from build123d import *

# Parameters (mm, degrees)
PAD_DEPTH = 10


with BuildPart() as part:
    # Sketch → Pad (new body)
    with BuildSketch(Plane.XY):
        with BuildLine():
            ThreePointArc((2.5, 0), (0, 2.5), (-2.5, 0))
            Line((-2.5, 0), (-2.5, -10))
            ThreePointArc((-2.5, -10), (0, -12.5), (2.5, -10))
            Line((2.5, -7.625), (2.5, -10))
            Line((7.5, -7.625), (2.5, -7.625))
            Line((7.5, -2.375), (7.5, -7.625))
            Line((2.5, -2.375), (7.5, -2.375))
            Line((2.5, 0), (2.5, -2.375))
        make_face()
    extrude(amount=PAD_DEPTH)


solid = part.part
Geometry: final body of the model. Coordinates: model frame, mm. A direction names the side the tool comes from. Give positions to 0.01 mm unless a question says otherwise; leave off trailing zeros. Write each loop counter-clockwise with the first axis right and the second up, starting at its lowest first coordinate (ties: lowest second). Pieces come first, ordered by that corner, then holes.
(1) First-contact query: P1, Ø2.5, axis at y = -1, z = 3.5, coming from the +X side; P2, Ø5.5, axis at x = 4, z = 4, coming from the -Y side; P3, Ø1, axis at y = 1, z = 3.5, coming from the -X side. Flat tips, straight axial feed; report the tip coordinate or a pass-through.
(2) Mould query, pull axis X, two halves, no side actions, for faces 4 (the flat face through (5, -2.375, 5)), 5 (the flat face through (2.5, -9, 5)), 6 (the cylindrical face through (0.1, 2.5, 4.9)). Classes: released by +X, released by -X, zero draft, split by the parting line, or undercut.
(3) Access query for faces 1 (the flat face through (5, -7.625, 5)), 2 (the flat face through (7.5, -5, 5)), 3 (the flat face through (2.5, -1, 5)). Directions: +Z, -Z, +X, -X, +Y, -Y. A direction counts if a zero-diameter tool reaches every point of the face in a straight line with its end or side. Return the directions, or none.
(4) Cut plane B-B, the plane y = -1. Return loops of the section in (x, z).
(5) Ray query, line 1 (Y direction, x = 3.5, z = 9) (3 decimals); line 2 (X direction, y = -8.75, z = 6.5); line 3 (Y direction, x = -0.25, z = 2). Return the intervals inside material, ascending.
(6) Cut plane C-C, the plane x = 6.25. Return loops of the section in (y, z) (3 decimals), then the cut area to 3 significant figures.
(7) Cut plane A-A, the plane z = 6.5. Return loops of the section in (x, y) (3 decimals), then the cut area to 3 significant figures.
Values follow:
1. P1: stops at x = 2.5
1. P2: stops at y = -12.17
1. P3: stops at x = -2.45
2. face 4: zero draft
2. face 5: released by +X
2. face 6: split by the parting line
3. face 1: +Z, -Z, +X, -Y
3. face 2: +Z, -Z, +X, +Y, -Y
3. face 3: +Z, -Z, +X, +Y
4. outline: (-2.5, 0) - (2.5, 0) - (2.5, 10) - (-2.5, 10) - close
5. line 1: y = -7.625 to -2.375
5. line 2: x = -2.5 to 2.5
5. line 3: y = -12.49 to 2.49
6. outline: (-7.625, 0) - (-2.375, 0) - (-2.375, 10) - (-7.625, 10) - close
6. area: 52.5 mm2
7. outline: (-2.5, -10) arc R2.5 ccw to (2.5, -10) - (2.5, -7.625) - (7.5, -7.625) - (7.5, -2.375) - (2.5, -2.375) - (2.5, 0) arc R2.5 ccw to (-2.5, 0) - close
7. area: 95.9 mm2
